from build123d import *

# Parameters (mm, degrees)
F1_DEPTH  = 22.6
F2_W      = 1
F2_H      = 10.5
F3_DEPTH  = 7.4
F4_W      = 7.4
F4_H      = 10.9
F5_DEPTH  = 1
F6_DEPTH  = 0.2
F7_W      = 3.9333333333
F7_H      = 8.7
F7_W_2    = 1.9666666667
F8_DEPTH  = 0.4
F9_SIZE   = 0.3
F11_DEPTH = 0.8
F13_W     = 1
F13_H     = 14.8
F14_DEPTH = 0.2
F15_W     = 3.9333333333
F15_H     = 6.5
F16_DEPTH = 0.2
F18_DEPTH = 0.25


with BuildPart() as f1:
    # F0 (on Right) → F1 (new body)
    with BuildSketch(Plane.YZ):
        Polygon((-6.2, 10.9), (-7.4, 10.9), (-7.4, 9.8), (-7, 9.8), (-7, 1.5), (-7.4, 1.5), (-7.4, 0.4), (-2.9, 0.4), (-2.9, 0), (-2, 0), (-2, 0.4), (0, 0.4), (0, 1.2), (-6.2, 1.2), align=None)
    extrude(amount=F1_DEPTH)

    # F2 (on face) → F3 (join, through all)
    with BuildSketch(Plane.XZ.offset(7.4)):
        with Locations((23.1, 5.65)):
            Rectangle(F2_W, F2_H)
    extrude(amount=-F3_DEPTH)

    # F4 (on face) → F5 (join)
    with BuildSketch(Plane(origin=(0, 0, 0), x_dir=(0, -1, 0), z_dir=(-1, 0, 0))):
        with Locations((3.7, 5.45)):
            Rectangle(F4_W, F4_H)
    extrude(amount=F5_DEPTH)

    # F6 (add): a face of the model
    f6_faces = [f1.faces().sort_by_distance(p)[0] for p in [
        (0, -3.1, 6.05),
    ]]
    extrude(f6_faces, amount=F6_DEPTH)

    # F7 (on face) → F8 (cut)
    with BuildSketch(Plane(origin=(-1, 0, 0), x_dir=(0, -1, 0), z_dir=(-1, 0, 0))):
        with Locations((4.5333333333, 5.45)):
            Rectangle(F7_W, F7_H)
        with Locations((0.9833333333, 5.45)):
            Rectangle(F7_W_2, F7_H)
    extrude(amount=-F8_DEPTH, mode=Mode.SUBTRACT)

    # F9
    f9_edges = [f1.edges().sort_by_distance(p)[0] for p in [
        (11.3, -7, 1.5),
        (11.3, -7, 9.8),
    ]]
    chamfer(f9_edges, length=F9_SIZE)

    # F10 (on face) → F11 (join)
    with BuildSketch(Plane(origin=(0, 0, 0), x_dir=(-1, 0, 0), z_dir=(0, 1, 0))):
        Polygon((-22.6, 9.5), (-22.6, 1.2), (-21.1, 1.2), (-22.3, 9.5), align=None)
    extrude(amount=-F11_DEPTH)

    # F12: F1 across face


with BuildPart() as f1_1:
    add(f1.part)
    add(f1.part.mirror(Plane(origin=(13.4187293548, 0, 3.5023232768), x_dir=(-1, 0, 0), z_dir=(0, 1, 0))))

    # F13 (on face) → F14 (join)
    with BuildSketch(Plane(origin=(0, 0, 0), x_dir=(1, 0, 0), z_dir=(0, 0, -1))):
        with Locations((-0.5, 0)):
            Rectangle(F13_W, F13_H)
    extrude(amount=F14_DEPTH)

    # F15 (on face) → F16 (join)
    with BuildSketch(Plane(origin=(-0.6, 0, 0), x_dir=(0, -1, 0), z_dir=(-1, 0, 0))):
        with Locations((0, 4.35)):
            Rectangle(F15_W, F15_H)
    extrude(amount=F16_DEPTH)

    # F17 (on face) → F18 (join)
    with BuildSketch(Plane(origin=(-0.8, 0, 0), x_dir=(0, -1, 0), z_dir=(-1, 0, 0))):
        Polygon((-0.7, 6.3), (-1, 6.3), (-1, 2.1), (1, 2.1), (1, 6.3), (0.7, 6.3), (0.7, 2.4), (-0.7, 2.4), align=None)
    extrude(amount=F18_DEPTH)


solid = f1_1.part
Check sheet for the modelled part. Datum: model origin and axes. Units: mm. A direction names the side the tool comes from. Round coordinates to 2 decimals unless told otherwise and drop trailing zeros. Write each loop counter-clockwise with the first axis right and the second up, starting at its lowest first coordinate (ties: lowest second). Pieces come first, ordered by that corner, then holes. Notation, with made-up numbers: (69.25, -28) -> (99.25, -28) arc R9 cw to (99.25, -22) -> close; hole circle Ø1 at (4, 60). An arc over 180 degrees is marked (long way). Answer as CSV lines item,"result". Start each with the question number.
1) Material ranges on line 1 (X direction, y = 2, z = 2.5); line 2 (Y direction, x = 11.25, z = 7); line 3 (X direction, y = 5.5, z = 2.5), recorded low to high. Write a range as from..to.
2) Section check B-B on x = 18.5. Enter the section's corners in (y, z), and give its area (3 significant figures).
3) Release check for a two-part mould opening along Y. For faces 4 (the flat face through (-0.8, 0, 4)), 5 (the flat face through (23.6, 0, 6)), 6 (the flat face through (10, -7.4, 1)) record: pulls with the +Y half, pulls with the -Y half, needs draft (parallel to the pull), parting line crosses it, or undercut.
4) Section check C-C on y = 3.75. Enter the section's corners in (x, z), and give its area (3 significant figures).
5) Go/stop test with flat-tipped pins: P1, Ø3, axis at x = 5.5, y = -2, coming from the +Z side; P2, Ø1, axis at x = 12, y = -2, coming from the -Z side; P3, Ø1.2, axis at x = 21.5, z = 5, coming from the +Y side. Record where each tip stops, or that it passes through.
6) Tool access check on faces 1 (the flat face through (11.5, 2.4, 0)), 2 (the flat face through (-0.6, 5, 6)), 3 (the flat face through (0.2, 0, 6)). Record the directions out of +Z, -Z, +X, -X, +Y, -Y that give a thin tool (end or side, any length) a straight path to the whole face; none if there is none.
Found:
1,line 1,"x = -1..0.2, 22.6..23.6"
1,line 2,"y = -7..-6.2, 6.2..7"
1,line 3,"x = -0.6..0.2, 22.6..23.6"
2,outline,"(-7.4, 0.4) -> (-2.9, 0.4) -> (-2.9, 0) -> (-2, 0) -> (-2, 0.4) -> (2, 0.4) -> (2, 0) -> (2.9, 0) -> (2.9, 0.4) -> (7.4, 0.4) -> (7.4, 1.5) -> (7.3, 1.5) -> (7, 1.8) -> (7, 9.5) -> (7.3, 9.8) -> (7.4, 9.8) -> (7.4, 10.9) -> (6.2, 10.9) -> (6.2, 1.2) -> (-6.2, 1.2) -> (-6.2, 10.9) -> (-7.4, 10.9) -> (-7.4, 9.8) -> (-7.3, 9.8) -> (-7, 9.5) -> (-7, 1.8) -> (-7.3, 1.5) -> (-7.4, 1.5) -> close"
2,area,"29.4 mm^2"
3,face 4,"undercut"
3,face 5,"needs draft"
3,face 6,"pulls with the -Y half"
4,outline,"(-1, -0.2) -> (0, -0.2) -> (0, 0.4) -> (23.6, 0.4) -> (23.6, 10.9) -> (22.6, 10.9) -> (22.6, 1.2) -> (0.2, 1.2) -> (0.2, 10.9) -> (-1, 10.9) -> (-1, 9.8) -> (-0.6, 9.8) -> (-0.6, 1.1) -> (-1, 1.1) -> close"
4,area,"38.1 mm^2"
5,P1,"stops at z = 1.2"
5,P2,"stops at z = 0"
5,P3,"stops at y = 7"
6,face 1,"-Z, +X, +Y, -Y"
6,face 2,"-X"
6,face 3,"+Z"
